Geometry check sheet. Reference: the model listing, model coordinates, mm. Face numbers are marked on the shaded views. A direction names the side the tool comes from. Give positions to 0.01 mm unless a question says otherwise; leave off trailing zeros. Write each loop counter-clockwise with the first axis right and the second up, starting at its lowest first coordinate (ties: lowest second). Pieces come first, ordered by that corner, then holes. Notation, with made-up numbers: (47.5, 54) -> (104.5, 54) arc R23 ccw to (104.5, 88) -> close; hole circle Ø11 at (-31.75, 76.5). An arc over 180 degrees is marked (long way). Use a Markdown table: item, result. Add a question column.
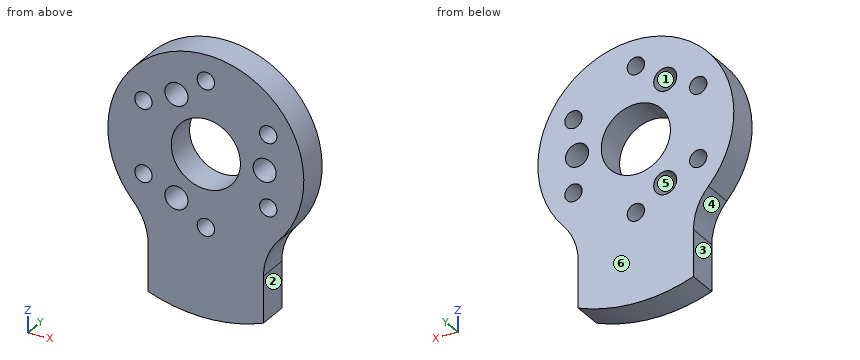
from build123d import *

# Parameters (mm, degrees)
SKETCH_1_R      = 2
SKETCH_1_R_2    = 1.5
SKETCH_1_R_3    = 6
EXTRUDE_1_DEPTH = 5.5
FILLET_1_R      = 10


with BuildPart() as part:
    # 草图1 → 凸台-拉伸1 (new body)
    with BuildSketch(Plane(origin=(0, 0, 0), x_dir=(1, 0, 0), z_dir=(0, 1, 0))):
        with BuildLine():
            Line((-10, 26.153393661), (-10, 13.747727085))
            ThreePointArc((-10, 13.747727085), (0, -17), (10, 13.747727085))
            Line((10, 13.747727085), (10, 26.153393661))
            ThreePointArc((10, 26.153393661), (0, 28), (-10, 26.153393661))
        make_face()
        with Locations(Location((-5.1, 8.833459119, 0), (0, 0, 270))):
            Circle(SKETCH_1_R, mode=Mode.SUBTRACT)
        with Locations(Location((-10.825317547, 6.25, 0), (0, 0, 270))):
            Circle(SKETCH_1_R_2, mode=Mode.SUBTRACT)
        with Locations(Location((10.2, 0, 0), (0, 0, 270))):
            Circle(SKETCH_1_R, mode=Mode.SUBTRACT)
        with Locations(Location((-5.1, -8.833459119, 0), (0, 0, 270))):
            Circle(SKETCH_1_R, mode=Mode.SUBTRACT)
        with Locations(Location((0, 12.5, 0), (0, 0, 270))):
            Circle(SKETCH_1_R_2, mode=Mode.SUBTRACT)
        with Locations(Location((10.825317547, 6.25, 0), (0, 0, 270))):
            Circle(SKETCH_1_R_2, mode=Mode.SUBTRACT)
        with Locations(Location((10.825317547, -6.25, 0), (0, 0, 270))):
            Circle(SKETCH_1_R_2, mode=Mode.SUBTRACT)
        with Locations(Location((0, -12.5, 0), (0, 0, 270))):
            Circle(SKETCH_1_R_2, mode=Mode.SUBTRACT)
        with Locations(Location((-10.825317547, -6.25, 0), (0, 0, 270))):
            Circle(SKETCH_1_R_2, mode=Mode.SUBTRACT)
        with Locations(Location((0, 0, 0), (0, 0, 270))):
            Circle(SKETCH_1_R_3, mode=Mode.SUBTRACT)
    extrude(amount=EXTRUDE_1_DEPTH)

    # 圆角1
    fillet_1_edges = [part.edges().sort_by_distance(p)[0] for p in [
        (10, 2.75, -13.747727085),
        (-10, 2.75, -13.747727085),
    ]]
    fillet(fillet_1_edges, radius=FILLET_1_R)


solid = part.part
1) Material ranges on probe 1 along X at (y, z) = (3, 0); probe 2 along X at (y, z) = (1.7, 1.5); probe 3 along Z at (x, y) = (12, 3.25), recorded low to high. Write a range as [from, to].
2) Sectioned sample at A-A, the plane z = 0. Enter the section's corners in (x, y).
3) Gauge pin test, flat end, axial feed: P1, Ø2, axis at x = -5.5, y = 4.5, coming from the -Z side. Record the tip position at first contact, or that the pin passes through.
4) Sectioned sample at C-C, the plane x = 2. Enter the section's corners in (y, z).
5) Tool access check on the marked faces 1, 2 and 3. Record the directions out of +Z, -Z, +X, -X, +Y, -Y that give a thin tool (end or side, any length) a straight path to the whole face; none if there is none.
6) Sectioned sample at B-B, the plane x = -5.1. Enter the section's corners in (y, z).
7) Draft check along Z on the marked faces 4, 5 and 6. Enter one of: +Z half, -Z half, draft (parallel to the pull), parting line (faces both ways), or undercut.
8) Sectioned sample at D-D, the plane y = 4.2. Count the separate pieces of the cut face and the enclosed holes in it, and give its area (3 significant figures).
Check values:
| question | item | result |
|---|---|---|
| 1 | probe 1 | [-17, -6], [6, 8.2], [12.2, 17] |
| 1 | probe 2 | [-16.93, -5.81], [5.81, 8.88], [11.52, 16.93] |
| 1 | probe 3 | [-12.14, -7.18], [-5.32, -0.87], [0.87, 5.32], [7.18, 12.04] |
| 2 | outline | (-17, 0) -> (-6, 0) -> (-6, 5.5) -> (-17, 5.5) -> close; (6, 0) -> (8.2, 0) -> (8.2, 5.5) -> (6, 5.5) -> close; (12.2, 0) -> (17, 0) -> (17, 5.5) -> (12.2, 5.5) -> close |
| 3 | P1 | z = -27.64 |
| 4 | outline | (0, -27.93) -> (5.5, -27.93) -> (5.5, -5.66) -> (0, -5.66) -> close; (0, 5.66) -> (5.5, 5.66) -> (5.5, 16.88) -> (0, 16.88) -> close |
| 5 | face 1 | +Y, -Y |
| 5 | face 2 | -Z, +X, +Y, -Y |
| 5 | face 3 | -Z, -X, +Y, -Y |
| 6 | outline | (0, -27.53) -> (5.5, -27.53) -> (5.5, -10.83) -> (0, -10.83) -> close; (0, -6.83) -> (5.5, -6.83) -> (5.5, -3.16) -> (0, -3.16) -> close; (0, 3.16) -> (5.5, 3.16) -> (5.5, 6.83) -> (0, 6.83) -> close; (0, 10.83) -> (5.5, 10.83) -> (5.5, 16.22) -> (0, 16.22) -> close |
| 7 | face 4 | -Z half |
| 7 | face 5 | undercut |
| 7 | face 6 | draft |
| 8 | separate pieces | 1 |
| 8 | enclosed holes | 10 |
| 8 | area | 948 mm² |
